For this review, take the finished solid that the model builds, in its own axes (mm). Face numbers are marked on the shaded views. A direction names the side the tool comes from. Give positions to 0.01 mm unless a question says otherwise; leave off trailing zeros. Order: outer loops, then holes, each group sorted by start corner. A loop starts at its lowest first (then second) coordinate and runs counter-clockwise, first axis right, second up. Notation, with made-up numbers: (27.25, 51) - (73.25, 51) arc R25 cw to (73.25, 86) - close; hole circle Ø6 at (9.25, 47.25). An arc over 180 degrees is marked (long way). One line per item, written item: value.
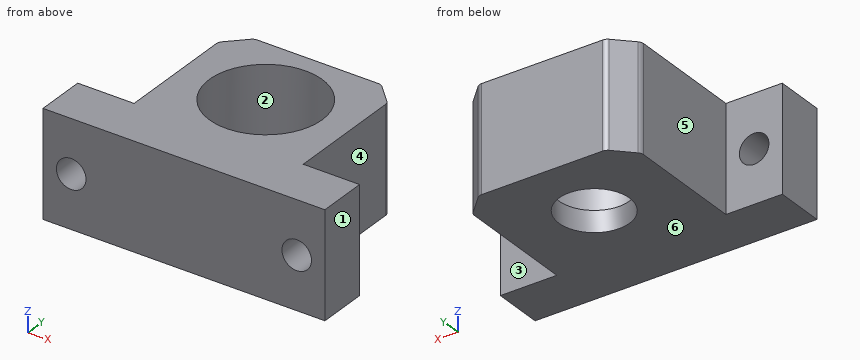
```python
from build123d import *

# Parameters (mm, degrees)
SKETCH1_R             = 8
BOSS_EXTRUDE1_DEPTH   = 15
CHAMFER1_SIZE         = 3
SKETCH2_R             = 8
SKETCH2_R_2           = 5
BOSS_EXTRUDE2_DEPTH   = 3
M5_TAPPED_HOLE1_D     = 4.2
M5_TAPPED_HOLE1_DEPTH = 103.56
M5_TAPPED_HOLE1_TIP   = 1.2618073
FILLET1_R             = 1


with BuildPart() as part:
    # Sketch1 → Boss-Extrude1 (new body)
    with BuildSketch(Plane.XY):
        Polygon((20, 0), (-20, 0), (-20, 7), (-12, 7), (-12, 27), (12, 27), (12, 7), (20, 7), align=None)
        with Locations((0, 16.5)):
            Circle(SKETCH1_R, mode=Mode.SUBTRACT)
    extrude(amount=BOSS_EXTRUDE1_DEPTH)

    # Chamfer1
    chamfer1_edges = [part.edges().sort_by_distance(p)[0] for p in [
        (-12, 27, 7.5),
        (12, 27, 7.5),
    ]]
    chamfer(chamfer1_edges, length=CHAMFER1_SIZE)

    # Sketch2 → Boss-Extrude2 (add)
    with BuildSketch(Plane(origin=(0, 0, 0), x_dir=(-1, 0, 0), z_dir=(0, 0, -1))):
        with Locations((0, 16.5)):
            Circle(SKETCH2_R)
        with Locations((0, 16.5)):
            Circle(SKETCH2_R_2, mode=Mode.SUBTRACT)
    extrude(amount=-BOSS_EXTRUDE2_DEPTH)

    # M5 Tapped Hole1
    with Locations(Plane(origin=(-16, 0, 7.5), x_dir=(0, 0, -1), z_dir=(0, -1, 0))):
        with Locations((0, 0), (0, 32)):
            Hole(M5_TAPPED_HOLE1_D / 2, depth=M5_TAPPED_HOLE1_DEPTH)
            with Locations((0, 0, -(M5_TAPPED_HOLE1_DEPTH + M5_TAPPED_HOLE1_TIP / 2))):  # 118° drill point
                Cone(0, M5_TAPPED_HOLE1_D / 2, M5_TAPPED_HOLE1_TIP, mode=Mode.SUBTRACT)

    # Fillet1
    fillet1_edges = [part.edges().sort_by_distance(p)[0] for p in [
        (-12, 24, 7.5),
        (9, 27, 7.5),
        (-9, 27, 7.5),
        (12, 24, 7.5),
    ]]
    fillet(fillet1_edges, radius=FILLET1_R)


solid = part.part
```
(1) Take a section at A-A (z = 7.5). Write out the cut boundary in (x, y), then the cut area to 3 significant figures.
Answers below:
outline: (-20, 0) - (-18.1, 0) - (-18.1, 7) - (-20, 7) - close; (-13.9, 0) - (13.9, 0) - (13.9, 7) - (12, 7) - (12, 23.59) arc R1 ccw to (11.71, 24.29) - (9.29, 26.71) arc R1 ccw to (8.59, 27) - (-8.59, 27) arc R1 ccw to (-9.29, 26.71) - (-11.71, 24.29) arc R1 ccw to (-12, 23.59) - (-12, 7) - (-13.9, 7) - close; (18.1, 0) - (20, 0) - (20, 7) - (18.1, 7) - close; hole circle Ø16 at (0, 16.5)
area: 491 mm^2
(2) Wall thickness on line 1 (X direction, y = 1.5, z = 7.5); line 2 (Y direction, x = 0, z = 6.25); line 3 (Y direction, x = 0, z = 1.45): over which ranges is each line inside the solid? List them lowest first. Write a range as from..to.
Answers below:
line 1: x = -20..-18.1, -13.9..13.9, 18.1..20
line 2: y = 0..8.5, 24.5..27
line 3: y = 0..11.5, 21.5..27
(3) Draft analysis for pull direction Y (two halves, no side actions). For the marked faces 1, 2 and 3, state which applies: pulls with the +Y half, pulls with the -Y half, needs draft (parallel to the pull), parting line crosses it, or undercut.
Answers below:
face 1: needs draft
face 2: undercut
face 3: pulls with the +Y half
(4) Take a section at B-B (x = 16). Write out the cut boundary in (y, z), then the cut area to 3 significant figures.
Answers below:
outline: (0, 0) - (7, 0) - (7, 5.4) - (0, 5.4) - close; (0, 9.6) - (7, 9.6) - (7, 15) - (0, 15) - close
area: 75.6 mm^2
(5) Take a section at C-C (y = 5). Write out the cut boundary in (x, z), then the cut area to 3 significant figures.
Answers below:
outline: (-20, 0) - (20, 0) - (20, 15) - (-20, 15) - close; hole circle Ø4.2 at (-16, 7.5); hole circle Ø4.2 at (16, 7.5)
area: 572 mm^2
(6) For P1, Ø2.5, axis at x = 14, z = 5, coming from the +Y side; P2, Ø8, axis at x = 0, y = 16.5, coming from the +Z side; P3, Ø14.5, axis at x = 0, y = 16.5, coming from the +Z side; P4, Ø9, axis at x = -15, z = 9.5, coming from the +Y side, all flat-tipped, find the tip position at first contact; note any pin that passes through.
Answers below:
P1: stops at y = 7
P2: passes through
P3: stops at z = 3
P4: stops at y = 25.5
(7) Machinability: for the marked faces 4, 5 and 6, which of the approach directions +Z, -Z, +X, -X, +Y, -Y give a long, thin tool a straight path to every point of the face, cutting with its end or side? Answer none if there is none.
Answers below:
face 4: +Z, -Z, +X, +Y
face 5: +Z, -Z, -X, +Y
face 6: -Z, +X, -X, +Y, -Y
(8) Take a section at D-D (y = 16.5). Write out the cut boundary in (x, z).
Answers below:
outline: (-12, 0) - (-5, 0) - (-5, 3) - (-8, 3) - (-8, 15) - (-12, 15) - close; (5, 0) - (12, 0) - (12, 15) - (8, 15) - (8, 3) - (5, 3) - close
